For this review, take the finished solid that the model builds, in its own axes (mm). Coordinates: 2 decimals unless noted, no trailing zeros.
1. To check wall thickness, follow probe 1 along Z at (x, y) = (-22, -106.5); probe 2 along Z at (x, y) = (12, -54). State the ranges of each line that lie inside material, in increasing order.
2. Take a section at A-A, the plane z = -24. Count the separate pieces of the cut face and the enclosed holes in it, then the cut area to 3 significant figures.
3. Clearance check with flat-ended pins moving along their axes: P1, Ø8.5, axis at x = -66.3, y = -107, coming from the +Z side; P2, Ø12.5, axis at x = -9.3, y = -50, coming from the +Z side. State where each tip first meets the part, or that it passes through.
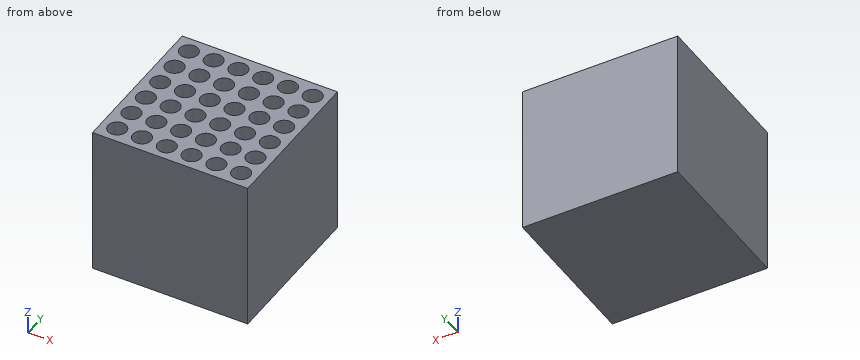
```python
from build123d import *

# Parameters (mm, degrees)
F0_W     = 119
F0_H     = 119
F1_DEPTH = 115
F2_D     = 14
F2_DEPTH = 110
F2_TIP   = 4.2060243332


with BuildPart() as f1:
    # F0 (on Top) → F1 (new body)
    with BuildSketch(Plane.XY):
        with Locations((-37.8049128657, -59.5)):
            Rectangle(F0_W, F0_H)
    extrude(amount=-F1_DEPTH)

    # F2
    with Locations(Plane.XY):
        with Locations((-85.3049128657, -12), (-66.3049128657, -12), (-47.3049128657, -12), (-28.3049128657, -12), (-9.3049128657, -12), (9.6950871343, -12), (9.6950871343, -31), (-9.3049128657, -31), (-28.3049128657, -31), (-47.3049128657, -31), (-66.3049128657, -31), (-85.3049128657, -31), (-85.3049128657, -50), (-66.3049128657, -50), (-47.3049128657, -50), (-28.3049128657, -50), (-9.3049128657, -50), (9.6950871343, -50), (9.6950871343, -69), (-9.3049128657, -69), (-28.3049128657, -69), (-47.3049128657, -69), (-66.3049128657, -69), (-85.3049128657, -69), (-85.3049128657, -88), (-66.3049128657, -88), (-47.3049128657, -88), (-28.3049128657, -88), (-9.3049128657, -88), (9.6950871343, -88), (9.6950871343, -107), (-9.3049128657, -107), (-28.3049128657, -107), (-47.3049128657, -107), (-66.3049128657, -107), (-85.3049128657, -107)):
            Hole(F2_D / 2, depth=F2_DEPTH)
            with Locations((0, 0, -(F2_DEPTH + F2_TIP / 2))):  # 118° drill point
                Cone(0, F2_D / 2, F2_TIP, mode=Mode.SUBTRACT)


solid = f1.part
```
Results list:
1. probe 1: z = -115 to -110.41
1. probe 2: z = -115 to -111.43
2. separate pieces: 1
2. enclosed holes: 36
2. area: 8,620 mm2
3. P1: stops at z = -111.65
3. P2: stops at z = -110.45
